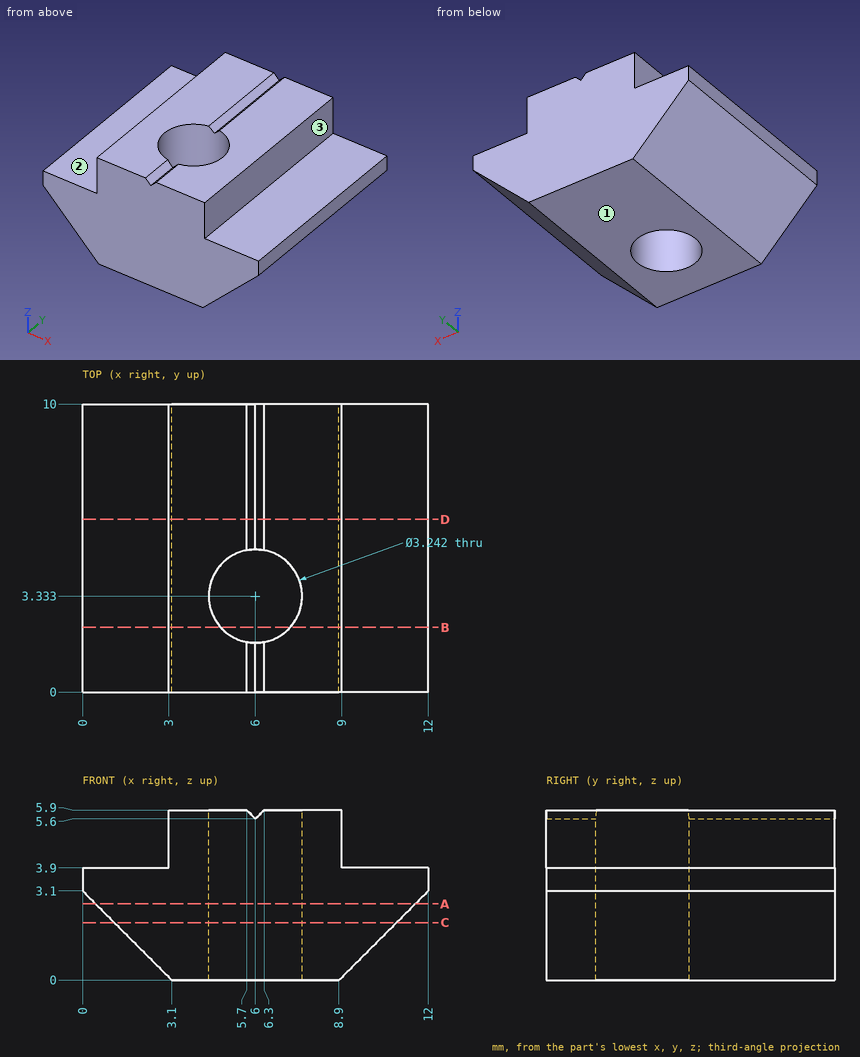
Here's the drawing with two shaded views (mm, measured from the low corner). I have some questions. A direction names the side the tool comes from. Round coordinates to 2 decimals unless told otherwise and drop trailing zeros. Loops run counter-clockwise (first coordinate to the right, second up) from the corner with the lowest first, then second, coordinate; pieces in that order, holes last.
Item 1: Which directions (+Z, -Z, +X, -X, +Y, -Y) give clear straight access to the entire face, cutting with the end or side of a thin tool? Please do the marked faces 1, 2 and 3.
Item 2: Suppose I cut it at A-A, the plane z = 2.65. Write out the boundary of the cut face in (x, y).
Item 3: Please list where these lines run through material, in increasing order: L1, parallel to X at y = 3.25, z = 3.75; L2, parallel to Y at x = 6, z = 2.45; L3, parallel to X at y = 1.25, z = 5.35.
Item 4: Suppose I cut it at D-D, the plane y = 6. Write out the boundary of the cut face in (x, z), then the cut area to 3 significant figures.
Item 5: Suppose I cut it at C-C, the plane z = 2. Write out the boundary of the cut face in (x, y).
Item 6: Will these pins go through, and if not, where does the flat tip stop? pin 1 Ø6 at (x, y) = (5.5, 4) entering from +Z; pin 2 Ø3.5 at (x, y) = (11, 3.5) entering from +Z; pin 3 Ø1 at (y, z) = (7, 5) entering from -X; pin 4 Ø0.6 at (y, z) = (5.5, 5.5) entering from +X.
Item 7: Suppose I cut it at B-B, the plane y = 2.25. Write out the boundary of the cut face in (x, z).
Reported:
1. face 1: -Z, +X, -X, +Y, -Y
1. face 2: +Z, -X, +Y, -Y
1. face 3: +Z, +X, +Y, -Y
2. outline: (0.45, 0) - (11.55, 0) - (11.55, 10) - (0.45, 10) - close; hole circle Ø3.24 at (6, 3.33)
3. L1: x = 0 to 4.38, 7.62 to 12
3. L2: y = 0 to 1.71, 4.95 to 10
3. L3: x = 3 to 9
4. outline: (0, 3.1) - (3.1, 0) - (8.9, 0) - (12, 3.1) - (12, 3.9) - (9, 3.9) - (9, 5.9) - (6.3, 5.9) - (6, 5.6) - (5.7, 5.9) - (3, 5.9) - (3, 3.9) - (0, 3.9) - close
4. area: 49.1 mm2
5. outline: (1.1, 0) - (10.9, 0) - (10.9, 10) - (1.1, 10) - close; hole circle Ø3.24 at (6, 3.33)
6. pin 1: stops at z = 5.9
6. pin 2: stops at z = 3.9
6. pin 3: stops at x = 3
6. pin 4: stops at x = 9
7. outline: (0, 3.1) - (3.1, 0) - (4.79, 0) - (4.79, 5.9) - (3, 5.9) - (3, 3.9) - (0, 3.9) - close; (7.21, 0) - (8.9, 0) - (12, 3.1) - (12, 3.9) - (9, 3.9) - (9, 5.9) - (7.21, 5.9) - close
